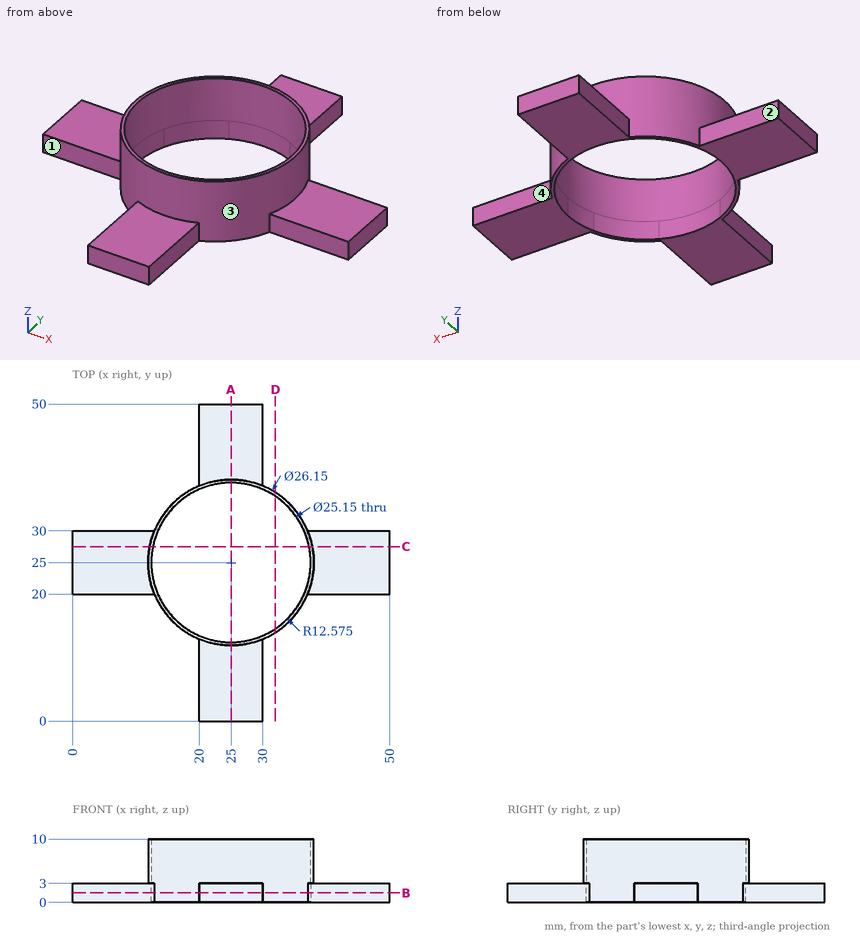
Here's the drawing with two shaded views (mm, measured from the low corner). I have some questions. A direction names the side the tool comes from. Coordinates: 2 decimals unless noted, no trailing zeros. Order: outer loops, then holes, each group sorted by start corner. A loop starts at its lowest first (then second) coordinate and runs counter-clockwise, first axis right, second up.
Q1. Will these pins go through, and if not, where does the flat tip stop? pin 1 (3.5 mm diameter, centred on y = 43.5, z = 1, fed in from +X); pin 2 (8 mm diameter, centred on x = 23.5, y = 46.5, fed in from +Z); pin 3 (1.5 mm diameter, centred on x = 45.5, z = 1, fed in from -Y).
Q2. Suppose I cut it at B-B on z = 1.5. Please give me the cut outline in (x, y) (3 decimals).
Q3. Which directions (+Z, -Z, +X, -X, +Y, -Y) give clear straight access to the entire face, cutting with the end or side of a thin tool? Please do the marked faces 1, 2, 3 and 4.
Q4. Suppose I cut it at C-C on y = 27.5. Please give me the cut outline in (x, z), and give its area (3 significant figures).
Q5. Please list where these lines run through material, in increasing order: L1, parallel to X at y = 25, z = 5 (3 decimals); L2, parallel to Y at x = 15.5, z = 1.
Q6. Suppose I cut it at D-D on x = 32. Please give me the cut outline in (y, z).
Q7. Suppose I cut it at A-A on x = 25. Please give me the cut outline in (y, z) (3 decimals), and give its area (4 significant figures).
Answer:
1. pin 1: stops at x = 30
1. pin 2: stops at z = 3
1. pin 3: stops at y = 20
2. outline: (0, 20) - (12.919, 20) arc R13.075 ccw to (20, 12.919) - (20, 0) - (30, 0) - (30, 12.919) arc R13.075 ccw to (37.081, 20) - (50, 20) - (50, 30) - (37.081, 30) arc R13.075 ccw to (30, 37.081) - (30, 50) - (20, 50) - (20, 37.081) arc R13.075 ccw to (12.919, 30) - (0, 30) - close; hole circle Ø25.15 at (25, 25)
3. face 1: +Z, -Z, -X, -Y
3. face 2: +Z, -Z, -X, +Y
3. face 3: +Z
3. face 4: +Z, -Z, +X, +Y
4. outline: (0, 0) - (12.68, 0) - (12.68, 10) - (12.17, 10) - (12.17, 3) - (0, 3) - close; (37.32, 0) - (50, 0) - (50, 3) - (37.83, 3) - (37.83, 10) - (37.32, 10) - close
4. area: 83.2 mm2
5. L1: x = 11.925 to 12.425, 37.575 to 38.075
5. L2: y = 16.02 to 16.76, 33.24 to 33.98
6. outline: (13.96, 0) - (14.55, 0) - (14.55, 10) - (13.96, 10) - close; (35.45, 0) - (36.04, 0) - (36.04, 10) - (35.45, 10) - close
7. outline: (0, 0) - (12.425, 0) - (12.425, 10) - (11.925, 10) - (11.925, 3) - (0, 3) - close; (37.575, 0) - (50, 0) - (50, 3) - (38.075, 3) - (38.075, 10) - (37.575, 10) - close
7. area: 81.55 mm2
